Verification items for the finished model (mm, model axes). A direction names the side the tool comes from. Coordinates: 2 decimals unless noted, no trailing zeros. Order: outer loops, then holes, each group sorted by start corner. A loop starts at its lowest first (then second) coordinate and runs counter-clockwise, first axis right, second up. Notation, with made-up numbers: M -3,57 L 39,57 A23 ccw 39,72 Z; hole C -18,76 d5. An arc over 180 degrees is marked long. Answer as a JSON object with one key per item and string values. Group by question number.
(1) Cross-section at A-A (y = -22.5). Enter the section's corners in (x, z), plus the area to 3 significant figures.
(2) Cross-section at B-B (z = 13). Enter the section's corners in (x, y).
(3) Access from +Z, -Z, +X, -X, +Y, -Y to the whole of each face (thin tool, end or side, straight path). Record for faces 5 (the face through (-53, -5.5, 11)), 6 (the face through (-53, -12, 21.893)), 7 (the face through (25.655, -22.021, 10.846)), 8 (the face through (-53, -12, 0.08)), 9 (the face through (-53, -18.5, 11)).
(4) Cross-section at C-C (x = 24.5). Enter the section's corners in (y, z), plus the area to 3 significant figures.
(5) Gauge pin test, flat ends, axial feed: pin 1 Ø11 at (x, z) = (-49.5, 15.5) entering from -Y; pin 2 Ø4 at (x, y) = (-59, -12.5) entering from +Z; pin 3 Ø11 at (x, z) = (-56.5, 11) entering from +Y. Record the tip position at first contact, or that the pin passes through.
(6) Mould release check, pull along X, two halves, no side actions. Record for faces 1 (the face through (42.5, 0, 11)), 2 (the face through (-38.49, -21.74, 10.85)), 3 (the face through (25.655, 22.979, 10.846)), 4 (the face through (-64.5, -12, 11)): released by +X, released by -X, zero draft, split by the parting line, or undercut.
(7) Cross-section at D-D (y = 20). Enter the section's corners in (x, z).
(8) Material ranges on line 1 (Y direction, x = 24.5, z = 16.25); line 2 (Y direction, x = -57.5, z = 17); line 3 (Z direction, x = -59.5, y = -14.5), recorded low to high.
Autodesk Fusion 360 part; units mm, degrees
sketch "Esquisse5" plane through (0, 0, 0) normal (0, 0, 1) x (1, 0, 0)
  line L0 (42.5, 26.5) -> (-42.5, 26.5)
  line L1 (-42.5, 26.5) -> (-42.5, -26.5)
  line L2 (-42.5, -26.5) -> (42.5, -26.5)
  line L3 (42.5, -26.5) -> (42.5, 26.5)
  circle A0 centre (-37.5, 22.5) radius 1.25
  circle A1 centre (24.5, 22.5) radius 1.25
  circle A2 centre (-37.5, -22.5) radius 1.25
  circle A3 centre (24.5, -22.5) radius 1.25
  dimension "d39" = 85
  dimension "d40" = 53
  dimension "d41" = 2.5
  dimension "d42" = 2.5
  dimension "d43" = 2.5
  dimension "d44" = 2.5
  dimension "d45" = 5
  dimension "d46" = 62
  dimension "d47" = 4
  dimension "d48" = 4
  dimension "d49" = 4
  dimension "d50" = 4
  dimension "d51" = 62
  dimension "d52" = 5
extrude "Extrusion10" add sketch "Esquisse5" along normal blind 22
sketch "Esquisse6" plane through (-42.5, 0, 0) normal (-1, 0, 0) x (0, -1, 0)
  line L0 (-26.5, 0) -> (26.5, 0)
  line L1 (26.5, 0) -> (26.5, 22)
  line L2 (26.5, 22) -> (-26.5, 22)
  line L3 (-26.5, 22) -> (-26.5, 0)
  line L4 (5.5, 21.893) -> (18.5, 21.893)
  line L5 (18.5, 21.893) -> (18.5, 0.0802)
  line L6 (18.5, 0.0802) -> (5.5, 0.0802)
  line L7 (5.5, 0.0802) -> (5.5, 21.893)
  dimension "d55" = 32
  dimension "d56" = 45
extrude "Extrusion11" add sketch "Esquisse6" along normal blind 22 contours L4 L5 L6 L7
Taken from the geometry:
{
 "1": {"outline": "M -42.5,0 L -38.75,0 L -38.75,22 L -42.5,22 Z; M -36.25,0 L 23.25,0 L 23.25,22 L -36.25,22 Z; M 25.75,0 L 42.5,0 L 42.5,22 L 25.75,22 Z", "area": "1,760 mm²"},
 "2": {"outline": "M -64.5,-18.5 L -42.5,-18.5 L -42.5,-26.5 L 42.5,-26.5 L 42.5,26.5 L -42.5,26.5 L -42.5,-5.5 L -64.5,-5.5 Z; hole C -37.5,-22.5 d2.5; hole C -37.5,22.5 d2.5; hole C 24.5,-22.5 d2.5; hole C 24.5,22.5 d2.5"},
 "3": {"face 5": "+Z, -Z, -X, +Y", "face 6": "+Z, -X, +Y, -Y", "face 7": "+Z, -Z", "face 8": "-Z, -X, +Y, -Y", "face 9": "+Z, -Z, -X, -Y"},
 "4": {"outline": "M -26.5,0 L -23.75,0 L -23.75,22 L -26.5,22 Z; M -21.25,0 L 21.25,0 L 21.25,22 L -21.25,22 Z; M 23.75,0 L 26.5,0 L 26.5,22 L 23.75,22 Z", "area": "1,060 mm²"},
 "5": {"pin 1": "stops at y = -18.5", "pin 2": "stops at z = 21.89", "pin 3": "stops at y = -5.5"},
 "6": {"face 1": "released by +X", "face 2": "undercut", "face 3": "undercut", "face 4": "released by -X"},
 "7": {"outline": "M -42.5,0 L 42.5,0 L 42.5,22 L -42.5,22 Z"},
 "8": {"line 1": "y = -26.5 to -23.75, -21.25 to 21.25, 23.75 to 26.5", "line 2": "y = -18.5 to -5.5", "line 3": "z = 0.08 to 21.89"}
}
